Geometry: final body of the model. Coordinates: model frame, mm. Face numbers are marked on the shaded views. A direction names the side the tool comes from. Give positions to 0.01 mm unless a question says otherwise; leave off trailing zeros. Order: outer loops, then holes, each group sorted by start corner. A loop starts at its lowest first (then second) coordinate and runs counter-clockwise, first axis right, second up. Notation, with made-up numbers: (61, 65.25) - (113, 65.25) arc R16 cw to (113, 92.25) - close; hole circle Ø10 at (-6.75, -33). An arc over 180 degrees is marked (long way). One line per question, with ' | ' between items. Start each with the question number.
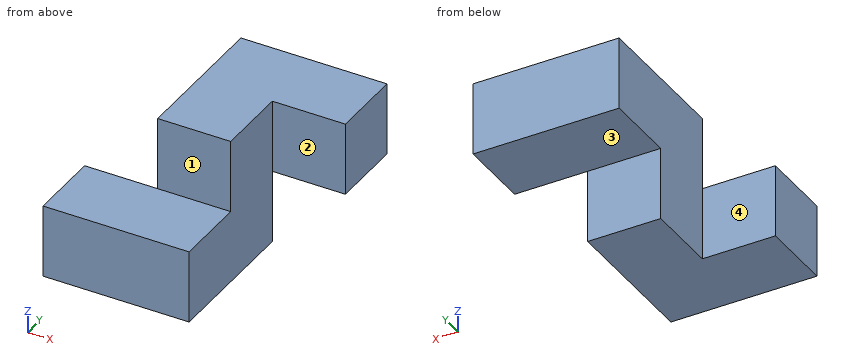
from build123d import *

# Parameters (mm, degrees)
F1_W      = 152.4
F1_H      = 76.2
F2_DEPTH  = 38.1
F3_W      = 76.2
F3_H      = 76.2
F4_DEPTH  = 76.2
F5_W      = 76.2
F5_H      = 76.2
F6_DEPTH  = 76.2
F7_W      = 76.2
F7_H      = 76.2
F8_DEPTH  = 76.2
F9_W      = 76.2
F9_H      = 76.2
F10_DEPTH = 76.2


# Not quite as in the source:
# - a variable given as a bare number and used for a length is read in inches; the dataset says mm whatever the document's units were


with BuildPart() as f2:
    # F1 (on Front) → F2 (new body, symmetric)
    with BuildSketch(Plane.XZ):
        Rectangle(F1_W, F1_H)
    extrude(amount=F2_DEPTH, both=True)

    # F3 (on face) → F4 (join)
    with BuildSketch(Plane(origin=(0, 38.1, 0), x_dir=(-1, 0, 0), z_dir=(0, 1, 0))):
        with Locations((-38.1, 0)):
            Rectangle(F3_W, F3_H)
    extrude(amount=F4_DEPTH)

    # F5 (on face) → F6 (join)
    with BuildSketch(Plane.XY.offset(38.1)):
        with Locations((38.1, 76.2)):
            Rectangle(F5_W, F5_H)
    extrude(amount=F6_DEPTH)

    # F7 (on face) → F8 (join)
    with BuildSketch(Plane(origin=(0, 114.3, 0), x_dir=(-1, 0, 0), z_dir=(0, 1, 0))):
        with Locations((-38.1, 76.2)):
            Rectangle(F7_W, F7_H)
    extrude(amount=F8_DEPTH)

    # F9 (on face) → F10 (join)
    with BuildSketch(Plane.YZ.offset(76.2)):
        with Locations((152.4, 76.2)):
            Rectangle(F9_W, F9_H)
    extrude(amount=F10_DEPTH)


solid = f2.part
(1) Cut plane D-D, the plane x = 128.5. Return the cut outline in (y, z), plus the area to 3 significant figures.
(2) Access query for the marked faces 1, 2, 3 and 4. Directions: +Z, -Z, +X, -X, +Y, -Y. A direction counts if a zero-diameter tool reaches every point of the face in a straight line with its end or side. Return the directions, or none.
(3) Cut plane B-B, the plane z = -4.5. Return the cut outline in (x, y).
(4) Cut plane A-A, the plane x = 32. Return the cut outline in (y, z), plus the area to 3 significant figures.
(5) Cut plane C-C, the plane y = 129.5. Return the cut outline in (x, z), plus the area to 3 significant figures.
(6) Material intervals for line 1 along Y through (x, z) = (-16.5, 29.5); line 2 along X through (y, z) = (-10.5, -15), sorted ascending. Write a range as from..to.
(7) Contact query for flat-ended pins moving along their axis: P1, Ø2, axis at y = 138, z = 62, coming from the -X side; P2, Ø23, axis at x = 100.5, z = 90, coming from the -Y side; P3, Ø1, axis at x = 126.5, y = 162.5, coming from the -Z side. Output: stop coordinate, or through.
Results are:
1) outline: (114.3, 38.1) - (190.5, 38.1) - (190.5, 114.3) - (114.3, 114.3) - close | area: 5,810 mm2
2) face 1: +Z, +X, -X, -Y | face 2: +Z, -Z, +X, -Y | face 3: -Z, +X, -X, +Y | face 4: +Z, -Z, -X, +Y
3) outline: (-76.2, -38.1) - (76.2, -38.1) - (76.2, 114.3) - (0, 114.3) - (0, 38.1) - (-76.2, 38.1) - close
4) outline: (-38.1, -38.1) - (114.3, -38.1) - (114.3, 38.1) - (190.5, 38.1) - (190.5, 114.3) - (38.1, 114.3) - (38.1, 38.1) - (-38.1, 38.1) - close | area: 23,200 mm2
5) outline: (0, 38.1) - (152.4, 38.1) - (152.4, 114.3) - (0, 114.3) - close | area: 11,600 mm2
6) line 1: -38.1..38.1 | line 2: -76.2..76.2
7) P1: x = 0 | P2: y = 114.3 | P3: z = 38.1
